from build123d import *

# Parameters (mm, degrees)
F0_R     = 82.55
F1_DEPTH = 25.4
F2_DEPTH = 25.4


with BuildPart() as f1:
    # F0 (on Top) → F1 (new body)
    with BuildSketch(Plane.XY):
        Circle(F0_R)
        with BuildLine():
            ThreePointArc((56.928029, 28.132713), (61.835183, 14.445071), (63.5, 0))
            ThreePointArc((63.5, 0), (63.321347, -4.759933), (62.786395, -9.493083))
            ThreePointArc((62.786395, -9.493083), (59.952025, -20.928562), (55.053901, -31.643609))
            ThreePointArc((55.053901, -31.643609), (47.94106, -41.640183), (39.038578, -50.082327))
            ThreePointArc((39.038578, -50.082327), (29.536178, -56.212669), (19.097084, -60.560312))
            ThreePointArc((19.097084, -60.560312), (6.547713, -63.161519), (-6.268377, -63.189852))
            ThreePointArc((-6.268377, -63.189852), (-19.387576, -60.467941), (-31.643609, -55.053901))
            ThreePointArc((-31.643609, -55.053901), (-44.901281, -44.901281), (-55.053901, -31.643609))
            ThreePointArc((-55.053901, -31.643609), (-61.35215, -16.375703), (-63.5, 0))
            ThreePointArc((-63.5, 0), (-62.421056, 11.655977), (-59.220888, 22.915855))
            ThreePointArc((-59.220888, 22.915855), (-50.972884, 37.868391), (-39.038578, 50.082327))
            ThreePointArc((-39.038578, 50.082327), (-26.536219, 57.689506), (-12.624355, 62.232433))
            ThreePointArc((-12.624355, 62.232433), (0, 63.5), (12.624355, 62.232433))
            ThreePointArc((12.624355, 62.232433), (28.894327, 56.545273), (43.035655, 46.692423))
            ThreePointArc((43.035655, 46.692423), (50.836013, 38.051935), (56.928029, 28.132713))
        make_face(mode=Mode.SUBTRACT)
    extrude(amount=F1_DEPTH)

    # F0 (on Top) → F2 (join)
    with BuildSketch(Plane.XY):
        with BuildLine():
            Line((-11.711573, 15.024698), (-39.038578, 50.082327))
            ThreePointArc((-39.038578, 50.082327), (-50.972884, 37.868391), (-59.220888, 22.915855))
            Line((-59.220888, 22.915855), (-17.766266, 6.874757))
            ThreePointArc((-17.766266, 6.874757), (-15.291865, 11.360517), (-11.711573, 15.024698))
        make_face()
        with BuildLine():
            Line((-19.05, 0), (-63.5, 0))
            ThreePointArc((-63.5, 0), (-61.35215, -16.375703), (-55.053901, -31.643609))
            Line((-55.053901, -31.643609), (-16.51617, -9.493083))
            ThreePointArc((-16.51617, -9.493083), (-18.405645, -4.912711), (-19.05, 0))
        make_face()
        with BuildLine():
            ThreePointArc((-31.643609, -55.053901), (-19.387576, -60.467941), (-6.268377, -63.189852))
            Line((-6.268377, -63.189852), (-1.880513, -18.956956))
            ThreePointArc((-1.880513, -18.956956), (-5.816273, -18.140382), (-9.493083, -16.51617))
            Line((-9.493083, -16.51617), (-31.643609, -55.053901))
        make_face()
        with BuildLine():
            ThreePointArc((19.097084, -60.560312), (29.536178, -56.212669), (39.038578, -50.082327))
            Line((39.038578, -50.082327), (11.711573, -15.024698))
            ThreePointArc((11.711573, -15.024698), (8.860853, -16.863801), (5.729125, -18.168094))
            Line((5.729125, -18.168094), (19.097084, -60.560312))
        make_face()
        with BuildLine():
            ThreePointArc((55.053901, -31.643609), (59.952025, -20.928562), (62.786395, -9.493083))
            Line((62.786395, -9.493083), (18.835918, -2.847925))
            ThreePointArc((18.835918, -2.847925), (17.985607, -6.278569), (16.51617, -9.493083))
            Line((16.51617, -9.493083), (55.053901, -31.643609))
        make_face()
        with BuildLine():
            Line((17.078409, 8.439814), (56.928029, 28.132713))
            ThreePointArc((56.928029, 28.132713), (50.836013, 38.051935), (43.035655, 46.692423))
            Line((43.035655, 46.692423), (12.910697, 14.007727))
            ThreePointArc((12.910697, 14.007727), (15.250804, 11.415581), (17.078409, 8.439814))
        make_face()
        with BuildLine():
            Line((3.787306, 18.66973), (12.624355, 62.232433))
            ThreePointArc((12.624355, 62.232433), (0, 63.5), (-12.624355, 62.232433))
            Line((-12.624355, 62.232433), (-3.787306, 18.66973))
            ThreePointArc((-3.787306, 18.66973), (0, 19.05), (3.787306, 18.66973))
        make_face()
        with BuildLine():
            ThreePointArc((19.05, 0), (18.550555, 4.333521), (17.078409, 8.439814))
            ThreePointArc((17.078409, 8.439814), (15.250804, 11.415581), (12.910697, 14.007727))
            ThreePointArc((12.910697, 14.007727), (8.668298, 16.963582), (3.787306, 18.66973))
            ThreePointArc((3.787306, 18.66973), (0, 19.05), (-3.787306, 18.66973))
            ThreePointArc((-3.787306, 18.66973), (-7.960866, 17.306852), (-11.711573, 15.024698))
            ThreePointArc((-11.711573, 15.024698), (-15.291865, 11.360517), (-17.766266, 6.874757))
            ThreePointArc((-17.766266, 6.874757), (-18.726317, 3.496793), (-19.05, 0))
            ThreePointArc((-19.05, 0), (-18.405645, -4.912711), (-16.51617, -9.493083))
            ThreePointArc((-16.51617, -9.493083), (-13.470384, -13.470384), (-9.493083, -16.51617))
            ThreePointArc((-9.493083, -16.51617), (-5.816273, -18.140382), (-1.880513, -18.956956))
            ThreePointArc((-1.880513, -18.956956), (1.964314, -18.948456), (5.729125, -18.168094))
            ThreePointArc((5.729125, -18.168094), (8.860853, -16.863801), (11.711573, -15.024698))
            ThreePointArc((11.711573, -15.024698), (14.382318, -12.492055), (16.51617, -9.493083))
            ThreePointArc((16.51617, -9.493083), (17.985607, -6.278569), (18.835918, -2.847925))
            ThreePointArc((18.835918, -2.847925), (18.996404, -1.42798), (19.05, 0))
        make_face()
    extrude(amount=F2_DEPTH)


solid = f1.part
Input: part model. Units: mm. Frame: model coordinates. Give positions to 0.01 mm unless a question says otherwise; leave off trailing zeros. Write each loop counter-clockwise with the first axis right and the second up, starting at its lowest first coordinate (ties: lowest second). Pieces come first, ordered by that corner, then holes. Notation, with made-up numbers: M -9.75,48 L 9.25,48 A13 ccw 9.25,69 Z; hole C 29.5,70.5 d2. An arc over 180 degrees is marked long. Use one line per item in the form item = value.
1. Cut plane C-C on y = 60. Return loops of the section in (x, z).
Outcome:
outline = M -56.7,0 L -20.79,0 L -20.79,25.4 L -56.7,25.4 Z; M -12.17,0 L 12.17,0 L 12.17,25.4 L -12.17,25.4 Z; M 20.79,0 L 56.7,0 L 56.7,25.4 L 20.79,25.4 Z
2. Ray query, L1, parallel to X at y = 28.5, z = 24.25; L2, parallel to X at y = -12.5, z = 8.75; L3, parallel to Y at x = -47.5, z = 7. Return the intervals inside material, ascending.
Outcome:
L1 = -77.47 to -22.22, -5.78 to 5.78, 26.27 to 77.47
L2 = -81.6 to -21.75, -14.38 to 14.38, 21.75 to 81.6
L3 = -67.51 to -42.14, -27.3 to 0, 18.38 to 67.51
3. First-contact query: P1, Ø12, axis at x = 21.5, z = 2.5, coming from the -Y side; P2, Ø3, axis at y = 2.5, z = 16.5, coming from the -X side; P3, Ø1.5, axis at y = -61, z = 15, coming from the -X side. Flat tips, straight axial feed; report the tip coordinate or a pass-through.
Outcome:
P1 = -81.08
P2 = -82.54
P3 = -56.43
4. Mould query, pull axis Y, two halves, no side actions, for faces 1 (the face through (-41, 0, 13)), 2 (the face through (-17.895, -80.587, 12.522)), 3 (the face through (-1, 1, 0)). Classes: released by +Y, released by -Y, zero draft, split by the parting line, or undercut.
Outcome:
face_1 = undercut
face_2 = split by the parting line
face_3 = zero draft
5. Cut plane B-B on z = 20.25. State how many separate pieces and enclosed holes the cut face has, and give its area (3 significant figures).
Outcome:
separate_pieces = 1
enclosed_holes = 7
area = 15,300 mm²
6. Cut plane D-D on y = -44. Return loops of the section in (x, z), and give its area (3 significant figures).
Outcome:
outline = M -69.85,0 L -45.78,0 L -45.78,25.4 L -69.85,25.4 Z; M -25.29,0 L -4.36,0 L -4.36,25.4 L -25.29,25.4 Z; M 13.87,0 L 34.3,0 L 34.3,25.4 L 13.87,25.4 Z; M 45.78,0 L 69.85,0 L 69.85,25.4 L 45.78,25.4 Z
area = 2,270 mm²
7. Cut plane A-A on x = 0. Return loops of the section in (y, z).
Outcome:
outline = M -82.55,0 L -63.5,0 L -63.5,25.4 L -82.55,25.4 Z; M -19.05,0 L 82.55,0 L 82.55,25.4 L -19.05,25.4 Z
